```python
from build123d import *

# Parameters (mm, degrees)
SKETCH2_W             = 65
SKETCH2_H             = 55
BOSS_EXTRUDE1_DEPTH   = 5
F_4_CLEARANCE_HOLE1_D = 3.2639


with BuildPart() as part:
    # Sketch2 → Boss-Extrude1 (new body)
    with BuildSketch(Plane(origin=(0, 0, 0), x_dir=(1, 0, 0), z_dir=(0, 1, 0))):
        Rectangle(SKETCH2_W, SKETCH2_H)
    extrude(amount=BOSS_EXTRUDE1_DEPTH)

    # #4 Clearance Hole1 (through all)
    with Locations(Plane(origin=(0, 0, 0), x_dir=(-1, 0, 0), z_dir=(0, -1, 0))):
        with Locations((-28.75, 15), (-15, 23.75), (15, 23.75), (28.75, 15), (28.75, -15), (15, -23.75), (-15, -23.75), (-28.75, -15)):
            Hole(F_4_CLEARANCE_HOLE1_D / 2)


solid = part.part
```
The model under review builds one solid part; all positions refer to its coordinate system, in mm. Round coordinates to 2 decimals unless told otherwise and drop trailing zeros. Loops run counter-clockwise (first coordinate to the right, second up) from the corner with the lowest first, then second, coordinate; pieces in that order, holes last. Notation, with made-up numbers: (89.25, 15) -> (95.25, 15) arc R19 ccw to (95.25, 21) -> close; hole circle Ø9 at (81, 46.25). An arc over 180 degrees is marked (long way). Answer as a JSON object with one key per item and string values. Group by question number.
1) We need section C-C on y = 3.55. Give the number of separate pieces and of enclosed holes in the cut face, then the cut area to 3 significant figures.
2) We need section B-B on z = 15. Write out the cut boundary in (x, y).
3) Mouldability with a two-part tool opening along X and no side actions: class faces 1 (the face through (14.646, 2.535, -22.157)), 2 (the face through (-32.5, 2, 0)), 3 (the face through (0, 2, 27.5)) as released by +X, released by -X, zero draft, split by the parting line, or undercut.
4) For line 1 (Z direction, x = 15, y = 3.4); line 2 (X direction, y = 2.2, z = 15); line 3 (Z direction, x = -28.75, y = 2.2), list the stretches that pass through material, from the lowest coordinate up. Write a range as [from, to].
5) For pin 1 Ø3 at (x, z) = (28.75, 15) entering from -Y, flat-tipped, find the tip position at first contact; note if it passes through.
6) We need section A-A on x = -15. Write out the cut boundary in (y, z).
Result set:
{
 "1": {"separate pieces": "1", "enclosed holes": "8", "area": "3,510 mm²"},
 "2": {"outline": "(-32.5, 0) -> (-30.38, 0) -> (-30.38, 5) -> (-32.5, 5) -> close; (-27.12, 0) -> (27.12, 0) -> (27.12, 5) -> (-27.12, 5) -> close; (30.38, 0) -> (32.5, 0) -> (32.5, 5) -> (30.38, 5) -> close"},
 "3": {"face 1": "undercut", "face 2": "released by -X", "face 3": "zero draft"},
 "4": {"line 1": "[-27.5, -25.38], [-22.12, 22.12], [25.38, 27.5]", "line 2": "[-32.5, -30.38], [-27.12, 27.12], [30.38, 32.5]", "line 3": "[-27.5, -16.63], [-13.37, 13.37], [16.63, 27.5]"},
 "5": {"pin 1": "through"},
 "6": {"outline": "(0, -27.5) -> (5, -27.5) -> (5, -25.38) -> (0, -25.38) -> close; (0, -22.12) -> (5, -22.12) -> (5, 22.12) -> (0, 22.12) -> close; (0, 25.38) -> (5, 25.38) -> (5, 27.5) -> (0, 27.5) -> close"}
}
